Input: part model. Units: mm. Frame: model coordinates. Give positions to 0.01 mm unless a question says otherwise; leave off trailing zeros. Order: outer loops, then holes, each group sorted by start corner. A loop starts at its lowest first (then second) coordinate and runs counter-clockwise, first axis right, second up. Notation, with made-up numbers: (-2.75, 80) - (51.25, 80) arc R13 cw to (51.25, 85) - close; hole circle Ø2 at (17, 15.25). An arc over 180 degrees is marked (long way). Answer in a Markdown table with one row per item. Add a question column.
1. Section query A-A on y = 4.5. Count the separate pieces of the cut face and the enclosed holes in it, and give its area (3 significant figures).
2. Section query B-B on x = 32. Return loops of the section in (y, z) (3 decimals), and give its area (3 significant figures).
3. Ray query, line 1 (X direction, y = 1.5, z = -6.35); line 2 (X direction, y = 4.25, z = 12) (1 decimal); line 3 (X direction, y = 5.25, z = 19). Return the intervals inside material, ascending. Write a range as [from, to].
4. Contact query for flat-ended pins moving along their axis: pin 1 (0.7 mm diameter, centred on x = 74, y = 3, fed in from -Z) (3 decimals); pin 2 (1.3 mm diameter, centred on y = 3, z = -23.5, fed in from +X); pin 3 (1.7 mm diameter, centred on y = 2, z = -23.5, fed in from -X). Output: stop coordinate, or through.
```python
from build123d import *

# Parameters (mm, degrees)
SKETCH1_W           = 428.625
SKETCH1_H           = 47.625
BOSS_EXTRUDE1_DEPTH = 6.35
SKETCH2_W           = 51.2445
SKETCH2_H           = 1.5875
SKETCH2_W_2         = 51.3715
CUT_EXTRUDE4_DEPTH  = 6.35
SKETCH4_W           = 3.175
SKETCH4_H           = 44.45
CUT_EXTRUDE5_DEPTH  = 6.35
SKETCH3_R           = 6.35
SKETCH3_W           = 12.7
SKETCH3_H           = 12.7
CUT_EXTRUDE6_DEPTH  = 6.35


with BuildPart() as part:
    # Sketch1 → Boss-Extrude1 (new body)
    with BuildSketch(Plane(origin=(0, 0, 0), x_dir=(1, 0, 0), z_dir=(0, 1, 0))):
        Rectangle(SKETCH1_W, SKETCH1_H)
    extrude(amount=BOSS_EXTRUDE1_DEPTH)

    # Sketch2 → Cut-Extrude4 (cut)
    with BuildSketch(Plane.XZ):
        Polygon((-124.841, -22.225), (-124.841, -23.8125), (-19.05, -23.8125), (-19.05, -22.225), (-70.45325, -22.225), (-73.31075, -22.225), align=None)
        with Locations((188.69025, 23.01875)):
            Rectangle(SKETCH2_W, SKETCH2_H)
        Polygon((19.05, 23.8125), (19.05, 22.225), (70.58025, 22.225), (73.43775, 22.225), (124.968, 22.225), (124.968, 23.8125), align=None)
        Polygon((-124.841, 22.225), (-73.31075, 22.225), (-70.45325, 22.225), (-19.05, 22.225), (-19.05, 23.8125), (-124.841, 23.8125), align=None)
        Polygon((19.05, -22.225), (19.05, -23.8125), (124.968, -23.8125), (124.968, -22.225), (73.43775, -22.225), (70.58025, -22.225), align=None)
        with Locations((188.69025, -23.01875)):
            Rectangle(SKETCH2_W, SKETCH2_H)
        with Locations((-188.62675, 23.01875)):
            Rectangle(SKETCH2_W_2, SKETCH2_H)
        with Locations((-188.62675, -23.01875)):
            Rectangle(SKETCH2_W_2, SKETCH2_H)
        Polygon((-70.45325, -4.445), (-70.45325, -10.795), (-69.088, -10.795), (-69.088, -14.605), (-70.45325, -14.605), (-70.45325, -22.225), (-73.31075, -22.225), (-73.31075, -14.605), (-74.676, -14.605), (-74.676, -10.795), (-73.31075, -10.795), (-73.31075, -4.445), align=None)
        Polygon((-70.45325, 4.445), (-73.31075, 4.445), (-73.31075, 10.795), (-74.676, 10.795), (-74.676, 14.605), (-73.31075, 14.605), (-73.31075, 22.225), (-70.45325, 22.225), (-70.45325, 14.605), (-69.088, 14.605), (-69.088, 10.795), (-70.45325, 10.795), align=None)
        Polygon((73.43775, 4.445), (70.58025, 4.445), (70.58025, 10.795), (69.215, 10.795), (69.215, 14.605), (70.58025, 14.605), (70.58025, 22.225), (73.43775, 22.225), (73.43775, 14.605), (74.803, 14.605), (74.803, 10.795), (73.43775, 10.795), align=None)
        Polygon((73.43775, -4.445), (73.43775, -10.795), (74.803, -10.795), (74.803, -14.605), (73.43775, -14.605), (73.43775, -22.225), (70.58025, -22.225), (70.58025, -14.605), (69.215, -14.605), (69.215, -10.795), (70.58025, -10.795), (70.58025, -4.445), align=None)
    extrude(amount=-CUT_EXTRUDE4_DEPTH, mode=Mode.SUBTRACT)

    # Sketch4 → Cut-Extrude5 (cut)
    with BuildSketch(Plane.XZ):
        with Locations((-212.725, 0)):
            Rectangle(SKETCH4_W, SKETCH4_H)
        with Locations((212.725, 0)):
            Rectangle(SKETCH4_W, SKETCH4_H)
    extrude(amount=-CUT_EXTRUDE5_DEPTH, mode=Mode.SUBTRACT)

    # Sketch3 → Cut-Extrude6 (cut)
    with BuildSketch(Plane.XZ):
        with Locations(Location((112.268, -6.35, 0), (0, 0, 270))):
            Circle(SKETCH3_R)
        with Locations((169.418, -6.35)):
            Rectangle(SKETCH3_W, SKETCH3_H)
    extrude(amount=-CUT_EXTRUDE6_DEPTH, mode=Mode.SUBTRACT)


solid = part.part
```
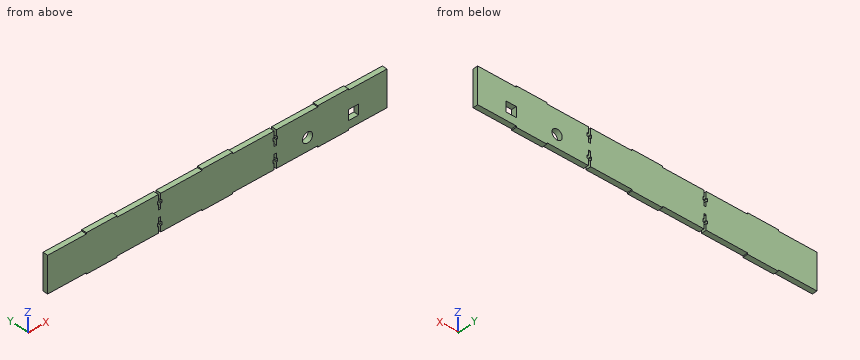
Answer:
| question | item | result |
|---|---|---|
| 1 | separate pieces | 1 |
| 1 | enclosed holes | 2 |
| 1 | area | 18,600 mm² |
| 2 | outline | (0, -22.225) - (6.35, -22.225) - (6.35, 22.225) - (0, 22.225) - close |
| 2 | area | 282 mm² |
| 3 | line 1 | x = [-211.14, -73.31], [-70.45, 70.58], [73.44, 105.92], [118.62, 163.07], [175.77, 211.14] |
| 3 | line 2 | x = [-211.1, -74.7], [-69.1, 69.2], [74.8, 211.1] |
| 3 | line 3 | x = [-211.14, -73.31], [-70.45, 70.58], [73.44, 211.14] |
| 4 | pin 1 | stops at z = -22.225 |
| 4 | pin 2 | stops at x = 163.07 |
| 4 | pin 3 | stops at x = -162.94 |
